Part model, mm, in its own coordinate system. Coordinates: 2 decimals unless noted, no trailing zeros. Write each loop counter-clockwise with the first axis right and the second up, starting at its lowest first coordinate (ties: lowest second). Pieces come first, ordered by that corner, then holes. Notation, with made-up numbers: M 69.5,9.5 L 106.5,9.5 A23 ccw 106.5,31.5 Z; hole C 43.5,87 d1. An arc over 180 degrees is marked long. Use a Markdown table: item, result. Add a question column.
Q1. Slice it at B-B on y = -5. Write the cut outline in (x, z).
Q2. Slice it at A-A on x = 13.5. Write the cut outline in (y, z), then the cut area to 3 significant figures.
Q3. Wall check: L1, parallel to X at y = 0, z = 0.55; L2, parallel to Y at x = 16, z = 1.6; L3, parallel to X at y = 12, z = 1.8. Give the ranges that are in metal, low to high. Write a range as from..to.
Q4. Slice it at C-C on z = 1.8. Write the cut outline in (x, y).
Q5. Pin check, flat tip, straight feed: pin 1 Ø6 at (x, y) = (-31.5, -2.5) entering from -Z. Stop position of the tip, or through.
from build123d import *

# Parameters (mm, degrees)
SKETCH_W     = 190
SKETCH_H     = 36
SKETCH_W_2   = 60
SKETCH_H_2   = 27
PAD_DEPTH    = 3
CHAMFER_SIZE = 10
FILLET_R     = 6


with BuildPart() as part:
    # Sketch → Pad (new body)
    with BuildSketch(Plane.XY):
        Rectangle(SKETCH_W, SKETCH_H)
        Rectangle(SKETCH_W_2, SKETCH_H_2, mode=Mode.SUBTRACT)
    extrude(amount=PAD_DEPTH)

    # Chamfer
    chamfer_edges = [part.edges().sort_by_distance(p)[0] for p in [
        (-95, -18, 1.5),
        (-95, 18, 1.5),
        (95, -18, 1.5),
        (95, 18, 1.5),
    ]]
    chamfer(chamfer_edges, length=CHAMFER_SIZE)

    # Fillet
    fillet_edges = [part.edges().sort_by_distance(p)[0] for p in [
        (-30, -13.5, 1.5),
        (-30, 13.5, 1.5),
        (30, 13.5, 1.5),
        (30, -13.5, 1.5),
    ]]
    fillet(fillet_edges, radius=FILLET_R)


solid = part.part
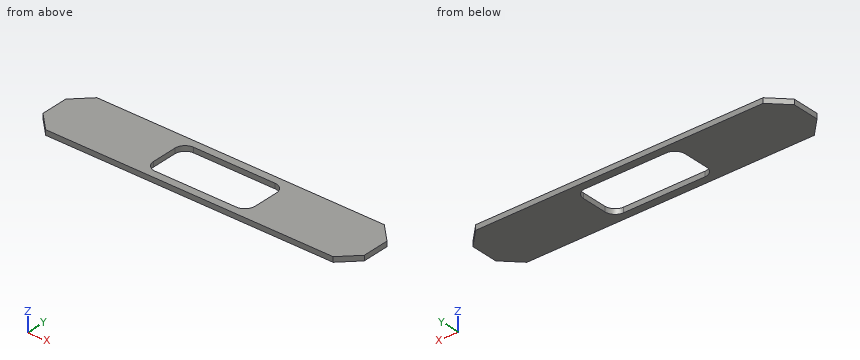
Recorded:
| question | item | result |
|---|---|---|
| 1 | outline | M -95,0 L -30,0 L -30,3 L -95,3 Z; M 30,0 L 95,0 L 95,3 L 30,3 Z |
| 2 | outline | M -18,0 L -13.5,0 L -13.5,3 L -18,3 Z; M 13.5,0 L 18,0 L 18,3 L 13.5,3 Z |
| 2 | area | 27.0 mm² |
| 3 | L1 | -95..-30, 30..95 |
| 3 | L2 | -18..-13.5, 13.5..18 |
| 3 | L3 | -91..-27.97, 27.97..91 |
| 4 | outline | M -95,-8 L -85,-18 L 85,-18 L 95,-8 L 95,8 L 85,18 L -85,18 L -95,8 Z; hole M -30,-7.5 A6 ccw -24,-13.5 L 24,-13.5 A6 ccw 30,-7.5 L 30,7.5 A6 ccw 24,13.5 L -24,13.5 A6 ccw -30,7.5 Z |
| 5 | pin 1 | z = 0 |
